Design review of the part built by this model. Coordinates are the model's own, in mm. A direction names the side the tool comes from. Give positions to 0.01 mm unless a question says otherwise; leave off trailing zeros. Loops run counter-clockwise (first coordinate to the right, second up) from the corner with the lowest first, then second, coordinate; pieces in that order, holes last. Notation, with made-up numbers: (-9, 74.25) - (4, 74.25) arc R25 ccw to (4, 88.25) - close; hole circle Ø9 at (74, 35.25). An arc over 180 degrees is marked (long way). Write each question's results on one line, items separated by ' | '.
from build123d import *

# Parameters (mm, degrees)
SKETCH_1_R      = 1.125
SKETCH_1_W      = 3
SKETCH_1_H      = 10
EXTRUDE_1_DEPTH = 3


with BuildPart() as part:
    # 草图1 → 凸台-拉伸1 (new body)
    with BuildSketch(Plane.XY):
        Polygon((40, 0), (40, 25), (0, 25), (0, 0), (2, 0), (5, 0), (7, 0), (7, -3), (15, -3), (15, 0), (25, 0), (25, -3), (33, -3), (33, 0), (35, 0), (38, 0), align=None)
        with Locations((10.7, 13)):
            Circle(SKETCH_1_R, mode=Mode.SUBTRACT)
        with Locations((29.3, 13)):
            Circle(SKETCH_1_R, mode=Mode.SUBTRACT)
        with Locations((3.5, 15)):
            Rectangle(SKETCH_1_W, SKETCH_1_H, mode=Mode.SUBTRACT)
        with Locations((36.5, 15)):
            Rectangle(SKETCH_1_W, SKETCH_1_H, mode=Mode.SUBTRACT)
        with Locations((20, 15)):
            Rectangle(SKETCH_1_W, SKETCH_1_H, mode=Mode.SUBTRACT)
    extrude(amount=EXTRUDE_1_DEPTH)


solid = part.part
(1) Take a section at A-A on x = 37. Give the boundary of the cut face in (y, z).
Answers below:
outline: (0, 0) - (10, 0) - (10, 3) - (0, 3) - close; (20, 0) - (25, 0) - (25, 3) - (20, 3) - close
(2) Tool access review of faces 1 (the flat face through (40, 12, 1)), 2 (the flat face through (33, -2, 1)), 3 (the flat face through (3, 20, 1)), 4 (the flat face through (20, 0, 1)), 5 (the flat face through (7, -1, 1)): name each direction out of +Z, -Z, +X, -X, +Y, -Y from which nothing blocks a thin tool from reaching the whole face with its end or side.
Answers below:
face 1: +Z, -Z, +X, +Y, -Y | face 2: +Z, -Z, +X, -Y | face 3: +Z, -Z | face 4: +Z, -Z, -Y | face 5: +Z, -Z, -X, -Y
(3) Take a section at B-B on y = 19.5. Give the boundary of the cut face in (x, z).
Answers below:
outline: (0, 0) - (2, 0) - (2, 3) - (0, 3) - close; (5, 0) - (18.5, 0) - (18.5, 3) - (5, 3) - close; (21.5, 0) - (35, 0) - (35, 3) - (21.5, 3) - close; (38, 0) - (40, 0) - (40, 3) - (38, 3) - close
(4) Take a section at C-C on z = 0.8. Give the boundary of the cut face in (x, y) (3 decimals), plus the area to 3 significant figures.
Answers below:
outline: (0, 0) - (7, 0) - (7, -3) - (15, -3) - (15, 0) - (25, 0) - (25, -3) - (33, -3) - (33, 0) - (40, 0) - (40, 25) - (0, 25) - close; hole (2, 10) - (5, 10) - (5, 20) - (2, 20) - close; hole circle Ø2.25 at (10.7, 13); hole (18.5, 10) - (21.5, 10) - (21.5, 20) - (18.5, 20) - close; hole circle Ø2.25 at (29.3, 13); hole (35, 10) - (38, 10) - (38, 20) - (35, 20) - close | area: 950 mm2
(5) Take a section at D-D on y = 13. Give the boundary of the cut face in (x, z) (3 decimals).
Answers below:
outline: (0, 0) - (2, 0) - (2, 3) - (0, 3) - close; (5, 0) - (9.575, 0) - (9.575, 3) - (5, 3) - close; (11.825, 0) - (18.5, 0) - (18.5, 3) - (11.825, 3) - close; (21.5, 0) - (28.175, 0) - (28.175, 3) - (21.5, 3) - close; (30.425, 0) - (35, 0) - (35, 3) - (30.425, 3) - close; (38, 0) - (40, 0) - (40, 3) - (38, 3) - close
(6) Wall thickness on line 1 along X through (y, z) = (11.5, 1.85); line 2 along Y through (x, z) = (10.7, 1.4) (3 decimals); line 3 along Y through (x, z) = (3, 0.6): over which ranges is each line inside the solid? List them lowest first. Write a range as from..to.
Answers below:
line 1: 0..2, 5..18.5, 21.5..35, 38..40 | line 2: -3..11.875, 14.125..25 | line 3: 0..10, 20..25
(7) Insertion check: P1, Ø0.9, axis at x = 20, z = 1.5, coming from the -Y side; P2, Ø0.9, axis at y = 15, z = 1.5, coming from the -X side. Each pin has a flat end and moves straight along its axis. Give the tip position at first contact, or say it passes through.
Answers below:
P1: y = 0 | P2: x = 0
